Work out the finished part from the listing and answer in its coordinate system (mm). Face numbers are marked on the shaded views. A direction names the side the tool comes from. Round coordinates to 2 decimals unless told otherwise and drop trailing zeros. Order: outer loops, then holes, each group sorted by start corner. A loop starts at its lowest first (then second) coordinate and runs counter-clockwise, first axis right, second up. Notation, with made-up numbers: (24.5, 0) - (62.5, 0) arc R27 cw to (62.5, 39) - close; hole circle Ø1 at (50.25, 7.5). An arc over 180 degrees is marked (long way). Use one line per item in the form item = value. Start each with the question number.
Q1. The part is cut by section A-A on z = 0. Determine the outline of the cut face in (x, y).
Q2. Find the intervals of material crossed by line 1 (Y direction, x = -10.75, z = 0); line 2 (X direction, y = 2, z = -2); line 3 (X direction, y = -1, z = 0.25), in increasing order. Write a range as [from, to].
Q3. The part is cut by section D-D on x = -8. Determine the outline of the cut face in (y, z), plus the area to 3 significant figures.
Q4. The part is cut by section C-C on y = 0.5. Determine the outline of the cut face in (x, z), plus the area to 3 significant figures.
Q5. The part is cut by section B-B on x = 38. Determine the outline of the cut face in (y, z).
Q6. Which of the six approach directions +Z, -Z, +X, -X, +Y, -Y give full straight-line access (tool end or side, diameter ignored) to the marked faces 1, 2 and 3?
Q7. Given P1, Ø1.5, axis at x = -6.5, y = -2.5, coming from the -Z side; P2, Ø1.2, axis at y = -0.5, z = -0.5, coming from the -X side; P3, Ø4, axis at x = 38, z = 0, coming from the -Y side, each flat-ended and moving along its own axis, determine where each tip first touches the part or whether it passes through.
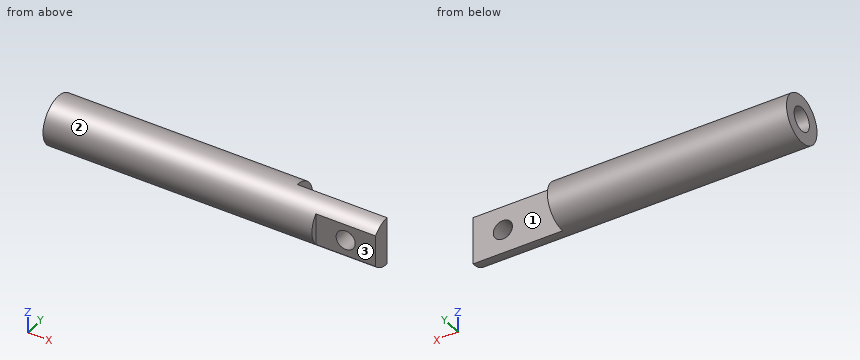
from build123d import *

# Parameters (mm, degrees)
CYLINDER026_R      = 2
CYLINDER026_DEPTH  = 5
CYLINDER035_R      = 1.6
CYLINDER035_DEPTH  = 5
BOX015001017_W     = 10
BOX015001017_H     = 10
BOX015001017_DEPTH = 10
BOX015001016_W     = 15
BOX015001016_H     = 10
BOX015001016_DEPTH = 10
CYLINDER025_R      = 4
CYLINDER025_DEPTH  = 55


with BuildPart() as cylinder036:
    # Cylinder026 → Cylinder026 (new body)
    with BuildSketch(Plane(origin=(-12, 0, 0), x_dir=(0, 0, -1), z_dir=(1, 0, 0))):
        Circle(CYLINDER026_R)
    extrude(amount=CYLINDER026_DEPTH)


with BuildPart() as cylinder035:
    # Cylinder035 → Cylinder035 (new body)
    with BuildSketch(Plane(origin=(38, -4, 0), x_dir=(1, 0, 0), z_dir=(0, 1, 0))):
        Circle(CYLINDER035_R)
    extrude(amount=CYLINDER035_DEPTH)


with BuildPart() as cube020:
    # Box015001017 → Box015001017 (new body)
    with BuildSketch(Plane(origin=(33, -13, -5), x_dir=(1, 0, 0), z_dir=(0, 0, 1))):
        with Locations((5, 5)):
            Rectangle(BOX015001017_W, BOX015001017_H)
    extrude(amount=BOX015001017_DEPTH)


with BuildPart() as cube019:
    # Box015001016 → Box015001016 (new body)
    with BuildSketch(Plane(origin=(28, 0, -5), x_dir=(1, 0, 0), z_dir=(0, 0, 1))):
        with Locations((7.5, 5)):
            Rectangle(BOX015001016_W, BOX015001016_H)
    extrude(amount=BOX015001016_DEPTH)


with BuildPart() as piston:
    # Cylinder025 → Cylinder025 (new body)
    with BuildSketch(Plane.ZY.offset(-43)):
        Circle(CYLINDER025_R)
    extrude(amount=CYLINDER025_DEPTH)

    # Cut004030: cut Cube019
    add(cube019.part, mode=Mode.SUBTRACT)

    # Cut001: cut Cube020
    add(cube020.part, mode=Mode.SUBTRACT)

    # Cut004028: cut Cylinder035
    add(cylinder035.part, mode=Mode.SUBTRACT)

    # Cut003: cut Cylinder036
    add(cylinder036.part, mode=Mode.SUBTRACT)


solid = piston.part
Found:
q1.outline = (-12, -4) - (33, -4) - (33, -3) - (36.4, -3) - (36.4, 0) - (28, 0) - (28, 4) - (-12, 4) - (-12, 2) - (-7, 2) - (-7, -2) - (-12, -2) - close; (39.6, -3) - (43, -3) - (43, 0) - (39.6, 0) - close
q2.line_1 = [-4, -2], [2, 4]
q2.line_2 = [-12, 28]
q2.line_3 = [-7, 36.42], [39.58, 43]
q3.outline = circle Ø8 at (0, 0); hole circle Ø4 at (0, 0)
q3.area = 37.7 mm²
q4.outline = (-12, -3.97) - (28, -3.97) - (28, 3.97) - (-12, 3.97) - (-12, 1.94) - (-7, 1.94) - (-7, -1.94) - (-12, -1.94) - close
q4.area = 298 mm²
q5.outline = (-3, -2.65) arc R4 ccw to (0, -4) - (0, -1.6) - (-3, -1.6) - close; (-3, 1.6) - (0, 1.6) - (0, 4) arc R4 ccw to (-3, 2.65) - close
q6.face_1 = +Z, -Z, +X, +Y
q6.face_2 = +X, -X
q6.face_3 = +Z, -Z, +X, -Y
q7.P1 = -3.6
q7.P2 = -7
q7.P3 = -3
